```python
from build123d import *

# Parameters (mm, degrees)
F0_R     = 17.5
F0_R_2   = 9.5
F1_DEPTH = 4.5
F2_R     = 16
F2_R_2   = 9.5
F3_DEPTH = 1.2
F4_R     = 17.5
F4_R_2   = 9.5
F5_DEPTH = 4.5
F6_SIZE  = 0.5


with BuildPart() as f1:
    # F0 (on Top) → F1 (new body)
    with BuildSketch(Plane.XY):
        Circle(F0_R)
        Circle(F0_R_2, mode=Mode.SUBTRACT)
    extrude(amount=F1_DEPTH)

    # F2 (on face) → F3 (join)
    with BuildSketch(Plane.XY.offset(4.5)):
        Circle(F2_R)
        Circle(F2_R_2, mode=Mode.SUBTRACT)
    extrude(amount=F3_DEPTH)

    # F4 (on face) → F5 (join)
    with BuildSketch(Plane.XY.offset(5.7)):
        Circle(F4_R)
        Circle(F4_R_2, mode=Mode.SUBTRACT)
    extrude(amount=F5_DEPTH)

    # F6
    f6_edges = [f1.edges().sort_by_distance(p)[0] for p in [
        (-17.5, 0, 10.2),
        (-17.5, 0, 0),
    ]]
    chamfer(f6_edges, length=F6_SIZE)


solid = f1.part
```
Source: CAD feature listing. Evaluate the final solid. Frame: model axes, mm. A direction names the side the tool comes from. Coordinates: 2 decimals unless noted, no trailing zeros. Write each loop counter-clockwise with the first axis right and the second up, starting at its lowest first coordinate (ties: lowest second). Pieces come first, ordered by that corner, then holes. Notation, with made-up numbers: M -20,67.25 L 17,67.25 A24 ccw 17,97.25 Z; hole C 54,-12 d9. An arc over 180 degrees is marked long. Answer as a JSON object with one key per item and string values.
1. Cut plane A-A on x = 0. Output: boundary loops of the cut face in (y, z), plus the area to 3 significant figures.
Evaluation:
{"outline": "M -17.5,0.5 L -17,0 L -9.5,0 L -9.5,10.2 L -17,10.2 L -17.5,9.7 L -17.5,5.7 L -16,5.7 L -16,4.5 L -17.5,4.5 Z; M 9.5,0 L 17,0 L 17.5,0.5 L 17.5,4.5 L 16,4.5 L 16,5.7 L 17.5,5.7 L 17.5,9.7 L 17,10.2 L 9.5,10.2 Z", "area": "159 mm^2"}
2. Access query for faces 1 (the cylindrical face through (-3.47, -15.62, 5.09)), 2 (the cylindrical face through (4.38, -8.43, 5.03)). Directions: +Z, -Z, +X, -X, +Y, -Y. A direction counts if a zero-diameter tool reaches every point of the face in a straight line with its end or side. Return the directions, or none.
Evaluation:
{"face 1": "none", "face 2": "+Z, -Z"}
3. Draft query along Z for faces 3 (the flat face through (7.7, -14.2, 4.5)), 4 (the cylindrical face through (-13.887, -10.648, 7.672)), 5 (the flat face through (7, -7, 10.2)). Return one class per face: released by +Z, released by -Z, zero draft, split by the parting line, or undercut.
Evaluation:
{"face 3": "undercut", "face 4": "zero draft", "face 5": "released by +Z"}
4. Cut plane C-C on z = 8.25. Output: boundary loops of the cut face in (x, y).
Evaluation:
{"outline": "C 0,0 d35; hole C 0,0 d19"}
5. Contact query for flat-ended pins moving along their axis: P1, Ø1.5, axis at x = -7.5, z = 5, coming from the +Y side; P2, Ø6, axis at y = -9, z = 4.5, coming from the -X side; P3, Ø17, axis at x = 0, y = 0, coming from the -Z side; P4, Ø2, axis at x = -4.5, z = 8, coming from the -Y side. Output: stop coordinate, or through.
Evaluation:
{"P1": "y = 16.06", "P2": "x = -16.44", "P3": "through", "P4": "y = -17.15"}
6. Ray query, L1, parallel to Z at x = 15, y = 7.5; L2, parallel to Y at x = 0, z = 6; L3, parallel to Y at x = -8, z = 3. Return the intervals inside material, ascending.
Evaluation:
{"L1": "0 to 4.5, 5.7 to 10.2", "L2": "-17.5 to -9.5, 9.5 to 17.5", "L3": "-15.56 to -5.12, 5.12 to 15.56"}
